from build123d import *

# Parameters (mm, degrees)
SKETCH1_R           = 18
BOSS_EXTRUDE1_DEPTH = 1.3
SKETCH2_R           = 14.75
BOSS_EXTRUDE2_DEPTH = 8.7
FILLET1_R           = 3
SKETCH3_R           = 13
CUT_EXTRUDE1_DEPTH  = 8.7
SKETCH4_R           = 2
BOSS_EXTRUDE3_DEPTH = 7
SKETCH5_R           = 1.15
CUT_EXTRUDE2_DEPTH  = 6
CUT_EXTRUDE3_DEPTH  = 5


with BuildPart() as part:
    # Sketch1 → Boss-Extrude1 (new body)
    with BuildSketch(Plane.XY):
        Circle(SKETCH1_R)
    extrude(amount=BOSS_EXTRUDE1_DEPTH)

    # Sketch2 → Boss-Extrude2 (add)
    with BuildSketch(Plane.XY.offset(1.3)):
        Circle(SKETCH2_R)
    extrude(amount=BOSS_EXTRUDE2_DEPTH)

    # Fillet1
    fillet1_edges = [part.edges().sort_by_distance(p)[0] for p in [
        (-14.75, 0, 10),
    ]]
    fillet(fillet1_edges, radius=FILLET1_R)

    # Sketch3 → Cut-Extrude1 (cut)
    with BuildSketch(Plane(origin=(0, 0, 0), x_dir=(-1, 0, 0), z_dir=(0, 0, -1))):
        Circle(SKETCH3_R)
    extrude(amount=-CUT_EXTRUDE1_DEPTH, mode=Mode.SUBTRACT)

    # Sketch4 → Boss-Extrude3 (add)
    with BuildSketch(Plane(origin=(0, 0, 8.7), x_dir=(-1, 0, 0), z_dir=(0, 0, -1))):
        Circle(SKETCH4_R)
    extrude(amount=BOSS_EXTRUDE3_DEPTH)

    # Sketch5 → Cut-Extrude2 (cut)
    with BuildSketch(Plane(origin=(0, 0, 1.7), x_dir=(-1, 0, 0), z_dir=(0, 0, -1))):
        Circle(SKETCH5_R)
    extrude(amount=-CUT_EXTRUDE2_DEPTH, mode=Mode.SUBTRACT)

    # Sketch8 → Cut-Extrude3 (cut)
    with BuildSketch(Plane.XY.offset(10)):
        with BuildLine():
            Line((-1.25, 5), (-1.25, 20))
            ThreePointArc((-1.25, 20), (0, 21.25), (1.25, 20))
            Line((1.25, 20), (1.25, 5))
            ThreePointArc((1.25, 5), (0, 3.75), (-1.25, 5))
        make_face()
        with BuildLine():
            Line((2.75, 5), (2.75, 20))
            ThreePointArc((2.75, 20), (4, 21.25), (5.25, 20))
            Line((5.25, 20), (5.25, 5))
            ThreePointArc((5.25, 5), (4, 3.75), (2.75, 5))
        make_face()
        with BuildLine():
            Line((6.75, 5), (6.75, 20))
            ThreePointArc((6.75, 20), (8, 21.25), (9.25, 20))
            Line((9.25, 20), (9.25, 5))
            ThreePointArc((9.25, 5), (8, 3.75), (6.75, 5))
        make_face()
        with BuildLine():
            Line((10.75, 5), (10.75, 20))
            ThreePointArc((10.75, 20), (12, 21.25), (13.25, 20))
            Line((13.25, 20), (13.25, 5))
            ThreePointArc((13.25, 5), (12, 3.75), (10.75, 5))
        make_face()
        with BuildLine():
            Line((-5.25, 5), (-5.25, 20))
            ThreePointArc((-5.25, 20), (-4, 21.25), (-2.75, 20))
            Line((-2.75, 20), (-2.75, 5))
            ThreePointArc((-2.75, 5), (-4, 3.75), (-5.25, 5))
        make_face()
        with BuildLine():
            Line((-9.25, 5), (-9.25, 20))
            ThreePointArc((-9.25, 20), (-8, 21.25), (-6.75, 20))
            Line((-6.75, 20), (-6.75, 5))
            ThreePointArc((-6.75, 5), (-8, 3.75), (-9.25, 5))
        make_face()
        with BuildLine():
            Line((-13.25, 5), (-13.25, 20))
            ThreePointArc((-13.25, 20), (-12, 21.25), (-10.75, 20))
            Line((-10.75, 20), (-10.75, 5))
            ThreePointArc((-10.75, 5), (-12, 3.75), (-13.25, 5))
        make_face()
    extrude(amount=-CUT_EXTRUDE3_DEPTH, mode=Mode.SUBTRACT)


solid = part.part
The listing builds one solid part. Answer for the finished solid, in the listing's coordinates (mm). A direction names the side the tool comes from. Round coordinates to 2 decimals unless told otherwise and drop trailing zeros. Order: outer loops, then holes, each group sorted by start corner. A loop starts at its lowest first (then second) coordinate and runs counter-clockwise, first axis right, second up. Notation, with made-up numbers: (7, 36.5) -> (28, 36.5) arc R21 ccw to (28, 53.5) -> close; hole circle Ø6 at (72.25, 64). An arc over 180 degrees is marked (long way). One line per item, written item: value.
Item 1: Straight lines are drawn through the part: L1, parallel to Y at x = 0, z = 6.55; L2, parallel to Y at x = 0, z = 2; L3, parallel to X at y = 13.5, z = 7.25. For each, find the intervals that lie inside material, in ascending order.
Taken from the geometry:
L1: y = -14.75 to -13, -2 to -1.15, 1.15 to 2
L2: y = -14.75 to -13, -2 to -1.15, 1.15 to 2, 13 to 14.75
L3: x = -5.92 to -5.25, -2.75 to -1.25, 1.25 to 2.75, 5.25 to 5.92
Item 2: For faces 1 (the cylindrical face through (-12.782, 4.025, 8.091)), 2 (the cylindrical face through (-2.343, 17.847, 0.641)), 3 (the cylindrical face through (10.316, -7.91, 4.289)), determine the directions among +Z, -Z, +X, -X, +Y, -Y from which every point of the face is accessible in a straight line to the end or side of a thin tool.
Taken from the geometry:
face 1: +Z, +Y
face 2: +Z, -Z
face 3: -Z
Item 3: Find section C-C, the plane y = 0. Give the vertices of the cut face in (x, z).
Taken from the geometry:
outline: (-18, 0) -> (-13, 0) -> (-13, 8.7) -> (-2, 8.7) -> (-2, 1.7) -> (-1.15, 1.7) -> (-1.15, 7.7) -> (1.15, 7.7) -> (1.15, 1.7) -> (2, 1.7) -> (2, 8.7) -> (13, 8.7) -> (13, 0) -> (18, 0) -> (18, 1.3) -> (14.75, 1.3) -> (14.75, 7) arc R3 ccw to (11.75, 10) -> (-11.75, 10) arc R3 ccw to (-14.75, 7) -> (-14.75, 1.3) -> (-18, 1.3) -> close
Item 4: Find section B-B, the plane z = 2.5. Give the vertices of the cut face in (x, y).
Taken from the geometry:
outline: circle Ø29.5 at (0, 0); circle Ø4 at (0, 0); hole circle Ø26 at (0, 0); hole circle Ø2.3 at (0, 0)
Item 5: Find section A-A, the plane x = 0. Give the vertices of the cut face in (y, z).
Taken from the geometry:
outline: (-18, 0) -> (-13, 0) -> (-13, 8.7) -> (-2, 8.7) -> (-2, 1.7) -> (-1.15, 1.7) -> (-1.15, 7.7) -> (1.15, 7.7) -> (1.15, 1.7) -> (2, 1.7) -> (2, 8.7) -> (3.75, 8.7) -> (3.75, 10) -> (-11.75, 10) arc R3 ccw to (-14.75, 7) -> (-14.75, 1.3) -> (-18, 1.3) -> close; (13, 0) -> (18, 0) -> (18, 1.3) -> (14.75, 1.3) -> (14.75, 5) -> (13, 5) -> close
Item 6: For a pull along X with two mould halves and no side action, classify faces 4 (the cylindrical face through (-3.2, -14.4, 4.1)), 5 (the flat face through (9.2, 9.4, 0)), 6 (the flat face through (-13.25, 6, 6)) as released by +X, released by -X, zero draft, split by the parting line, or undercut.
Taken from the geometry:
face 4: split by the parting line
face 5: zero draft
face 6: undercut
Item 7: Given P1, Ø1, axis at x = -9.5, z = 4.5, coming from the +Y side; P2, Ø21, axis at x = 0, y = 0, coming from the -Z side; P3, Ø0.8, axis at x = 4, y = 13.5, coming from the +Z side, each flat-ended and moving along its own axis, determine where each tip first touches the part or whether it passes through.
Taken from the geometry:
P1: stops at y = 11.69
P2: stops at z = 1.7
P3: stops at z = 5
